For this review, use the dimensioned drawing (mm, ordinates from the lowest corner) and the shaded views. A direction names the side the tool comes from. Round coordinates to 2 decimals unless told otherwise and drop trailing zeros. Loops run counter-clockwise (first coordinate to the right, second up) from the corner with the lowest first, then second, coordinate; pieces in that order, holes last. Notation, with made-up numbers: (-14.5, -2.5) - (26.5, -2.5) arc R33 ccw to (26.5, 25.5) - close; hole circle Ø4 at (16, 45). An arc over 180 degrees is marked (long way). Return JSON: item names as keys, results as strings. Group by question number.
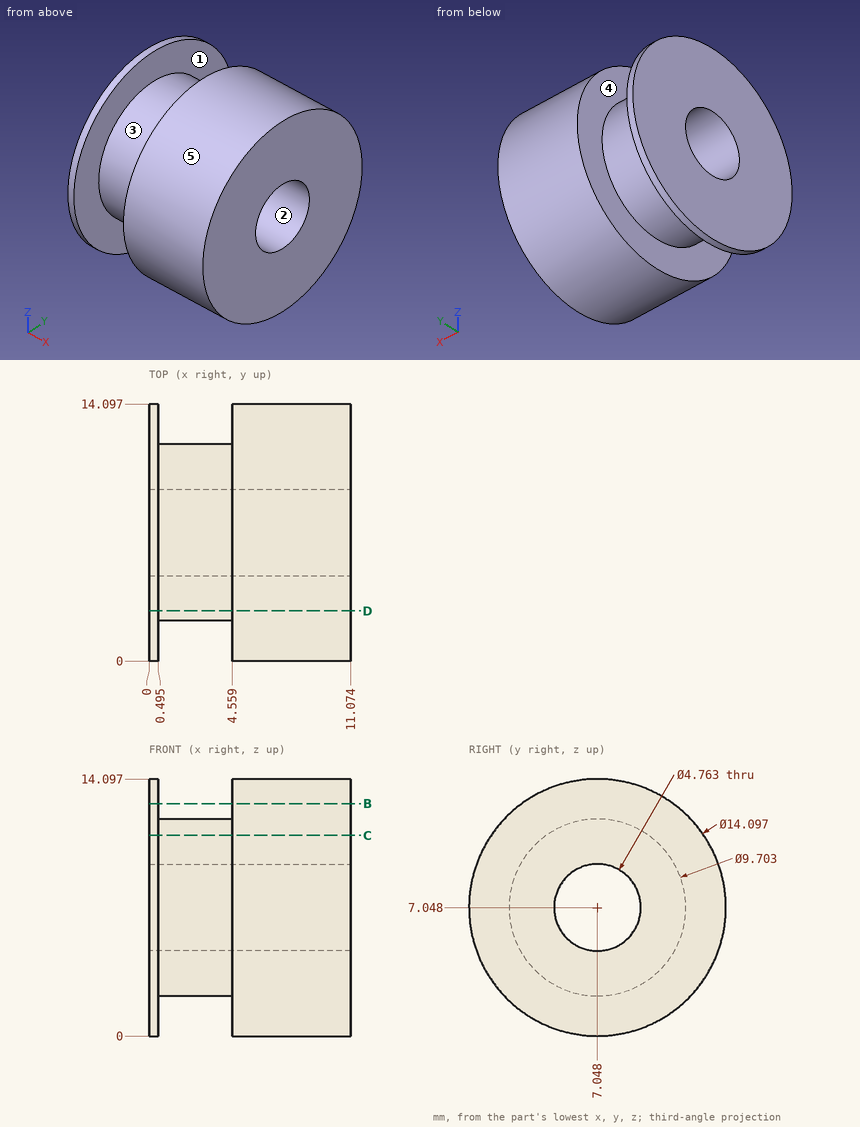
Q1. Insertion check: pin 1 Ø5 at (x, z) = (4.5, 2) entering from -Y; pin 2 Ø1.5 at (x, z) = (8, 4) entering from -Y (1 decimal). Each pin has a flat end and moves straight along its axis. Give the tip position at first contact, or say it passes through.
Q2. Draft analysis for pull direction Y (two halves, no side actions). For the marked faces 1, 2 and 3, state which applies: pulls with the +Y half, pulls with the -Y half, needs draft (parallel to the pull), parting line crosses it, or undercut.
Q3. Add section C-C, the plane z = 11. State the section outline as (x, y) points (1 decimal).
Q4. Tool access review of the marked faces 4 and 5: name each direction out of +Z, -Z, +X, -X, +Y, -Y from which nothing blocks a thin tool from reaching the whole face with its end or side.
Q5. For line 1 (X direction, y = 12.25, z = 6.75) (1 decimal); line 2 (Z direction, x = 8, y = 6) (1 decimal); line 3 (Z direction, x = 1, y = 9) (1 decimal), list the stretches that pass through material, from the lowest coordinate up.
Q6. Add section B-B, the plane z = 12.75. State the section outline as (x, y) points (1 decimal).
Q7. Add section D-D, the plane y = 2.75. State the section outline as (x, z) points (1 decimal).
Evaluation:
{
 "1": {"pin 1": "y = 0.48", "pin 2": "y = 0.4"},
 "2": {"face 1": "needs draft", "face 2": "undercut", "face 3": "parting line crosses it"},
 "3": {"outline": "(0, 1.2) - (0.5, 1.2) - (0.5, 4.2) - (4.6, 4.2) - (4.6, 1.2) - (11.1, 1.2) - (11.1, 12.9) - (4.6, 12.9) - (4.6, 9.9) - (0.5, 9.9) - (0.5, 12.9) - (0, 12.9) - close"},
 "4": {"face 4": "none", "face 5": "+X, -X"},
 "5": {"line 1": "0 to 0.5, 4.6 to 11.1", "line 2": "0.1 to 4.9, 9.2 to 14", "line 3": "2.6 to 5.7, 8.4 to 11.5"},
 "6": {"outline": "(0, 2.9) - (0.5, 2.9) - (0.5, 11.2) - (0, 11.2) - close; (4.6, 2.9) - (11.1, 2.9) - (11.1, 11.2) - (4.6, 11.2) - close"},
 "7": {"outline": "(0, 1.5) - (0.5, 1.5) - (0.5, 4.8) - (4.6, 4.8) - (4.6, 1.5) - (11.1, 1.5) - (11.1, 12.6) - (4.6, 12.6) - (4.6, 9.3) - (0.5, 9.3) - (0.5, 12.6) - (0, 12.6) - close"}
}
